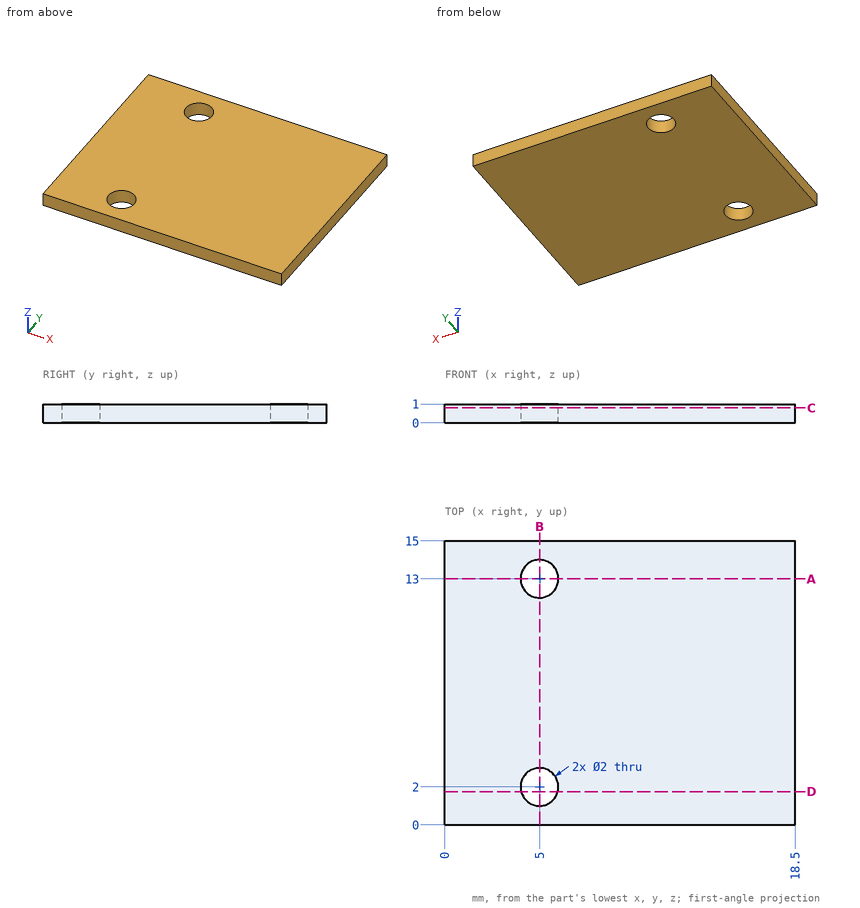
Geometry check sheet. Reference: drawing and pictorial views, mm from the part's lowest x, y, z. Round coordinates to 2 decimals unless told otherwise and drop trailing zeros. Loops run counter-clockwise (first coordinate to the right, second up) from the corner with the lowest first, then second, coordinate; pieces in that order, holes last. Notation, with made-up numbers: (85.5, 68.25) - (128.5, 68.25) arc R22 cw to (128.5, 96.25) - close; hole circle Ø3 at (-13, 82). An arc over 180 degrees is marked (long way). Answer as CSV lines item,"result".
(1) Material ranges on line 1 along Y through (x, z) = (5, 0.6); line 2 along X through (y, z) = (12.25, 0.9); line 3 along X through (y, z) = (12.5, 0.5), recorded low to high.
Output values:
line 1,"y = 0 to 1, 3 to 12, 14 to 15"
line 2,"x = 0 to 4.34, 5.66 to 18.5"
line 3,"x = 0 to 4.13, 5.87 to 18.5"
(2) Cross-section at A-A, the plane y = 13. Enter the section's corners in (x, z), and give its area (3 significant figures).
Output values:
outline,"(0, 0) - (4, 0) - (4, 1) - (0, 1) - close; (6, 0) - (18.5, 0) - (18.5, 1) - (6, 1) - close"
area,"16.5 mm²"
(3) Cross-section at B-B, the plane x = 5. Enter the section's corners in (y, z).
Output values:
outline,"(0, 0) - (1, 0) - (1, 1) - (0, 1) - close; (3, 0) - (12, 0) - (12, 1) - (3, 1) - close; (14, 0) - (15, 0) - (15, 1) - (14, 1) - close"
(4) Cross-section at D-D, the plane y = 1.75. Enter the section's corners in (x, z).
Output values:
outline,"(0, 0) - (4.03, 0) - (4.03, 1) - (0, 1) - close; (5.97, 0) - (18.5, 0) - (18.5, 1) - (5.97, 1) - close"
(5) Cross-section at C-C, the plane z = 0.8. Enter the section's corners in (x, y).
Output values:
outline,"(0, 0) - (18.5, 0) - (18.5, 15) - (0, 15) - close; hole circle Ø2 at (5, 2); hole circle Ø2 at (5, 13)"
